```python
from build123d import *

# Parameters (mm, degrees)
SKETCH1_W          = 55
SKETCH1_H          = 55
BASE_FLANGE1_DEPTH = 0.7
EDGE_FLANGE1_DEPTH = 55
SKETCH10_R         = 2
CUT_EXTRUDE1_DEPTH = 10


# Sheet-metal steps are written as plain solids
with BuildPart() as part:
    # Sketch1 → Base-Flange1 (new body)
    with BuildSketch(Plane.XY):
        Rectangle(SKETCH1_W, SKETCH1_H)
    extrude(amount=-BASE_FLANGE1_DEPTH)

    # Edge-Flange1 section (across the edge) → Edge-Flange1 (add)
    with BuildSketch(Plane(origin=(-27.5, 27.914213562, -0.7), x_dir=(0, -0.7071067811865438, -0.7071067811865512), z_dir=(1, 0, 0))):
        with BuildLine():
            Line((-0.7, 0.414213562), (-0.7, 54.710050506))
            Line((-0.7, 54.710050506), (0, 54.710050506))
            Line((0, 54.710050506), (0, 0.414213562))
            ThreePointArc((0, 0.414213562), (0.076120467, 0.03153013), (0.292893219, -0.292893219))
            Line((0.292893219, -0.292893219), (-0.202081528, -0.787867966))
            ThreePointArc((-0.202081528, -0.787867966), (-0.570595205, -0.236348273), (-0.7, 0.414213562))
        make_face()
    extrude(amount=EDGE_FLANGE1_DEPTH)

    # Sketch10 → Cut-Extrude1 (cut)
    with BuildSketch(Plane.XY):
        Circle(SKETCH10_R)
    extrude(amount=-CUT_EXTRUDE1_DEPTH, mode=Mode.SUBTRACT)


solid = part.part
```
Verification items for the finished model (mm, model axes). A direction names the side the tool comes from. Coordinates: 2 decimals unless noted, no trailing zeros. Loops run counter-clockwise (first coordinate to the right, second up) from the corner with the lowest first, then second, coordinate; pieces in that order, holes last. Notation, with made-up numbers: (83, 0.25) -> (111, 0.25) arc R26 ccw to (111, 19.25) -> close; hole circle Ø5 at (-24.75, -26). An arc over 180 degrees is marked (long way). Answer in a Markdown table with one row per item. Add a question column.
1. Section check B-B, the plane x = 0. Enter the section's corners in (y, z), then the cut area to 3 significant figures.
2. Draft check along Y on faces 3 (the face through (-0.434, -1.952, -0.345)), 4 (the face through (-0.385, 47.672, -20.458)), 5 (the face through (-0.385, 47.63, -19.426)). Enter one of: +Y half, -Y half, draft (parallel to the pull), parting line (faces both ways), or undercut.
3. Section check D-D, the plane y = 12.5. Enter the section's corners in (x, z), then the cut area to 3 significant figures.
4. Access from +Z, -Z, +X, -X, +Y, -Y to the whole of each face (thin tool, end or side, straight path). Record for faces 1 (the face through (0, 6, 0)), 2 (the face through (0, 6, -0.7)).
5. Depth check by flat-ended pin: P1, Ø10, axis at x = 6.5, y = 31.5, coming from the -Z side; P2, Ø6, axis at x = 4, z = -12, coming from the -Y side; P3, Ø1, axis at x = 7.5, y = -14, coming from the -Z side. Enter the tip coordinate at first touch or a pass-through.
6. Section check A-A, the plane y = 0. Enter the section's corners in (x, z).
7. Section check C-C, the plane x = 20.5. Enter the section's corners in (y, z).
8. Material ranges on probe 1 along Y at (x, z) = (0, -0.5); probe 2 along Z at (x, y) = (-22, -11.5); probe 3 along Y at (x, z) = (0, -0.2), recorded low to high. Write a range as [from, to].
Derived:
| question | item | result |
|---|---|---|
| 1 | outline | (-27.5, -0.7) -> (-2, -0.7) -> (-2, 0) -> (-27.5, 0) -> close; (2, -0.7) -> (27.5, -0.7) arc R1 cw to (28.21, -0.99) -> (66.6, -39.39) -> (67.1, -38.89) -> (28.7, -0.5) arc R1.7 ccw to (27.5, 0) -> (2, 0) -> close |
| 1 | area | 74.4 mm² |
| 2 | face 3 | undercut |
| 2 | face 4 | -Y half |
| 2 | face 5 | +Y half |
| 3 | outline | (-27.5, -0.7) -> (27.5, -0.7) -> (27.5, 0) -> (-27.5, 0) -> close |
| 3 | area | 38.5 mm² |
| 4 | face 1 | +Z, +X, -X, +Y, -Y |
| 4 | face 2 | -Z, +X, -X, -Y |
| 5 | P1 | stops at z = -9.29 |
| 5 | P2 | stops at y = 36.21 |
| 5 | P3 | stops at z = -0.7 |
| 6 | outline | (-27.5, -0.7) -> (-2, -0.7) -> (-2, 0) -> (-27.5, 0) -> close; (2, -0.7) -> (27.5, -0.7) -> (27.5, 0) -> (2, 0) -> close |
| 7 | outline | (-27.5, -0.7) -> (27.5, -0.7) arc R1 cw to (28.21, -0.99) -> (66.6, -39.39) -> (67.1, -38.89) -> (28.7, -0.5) arc R1.7 ccw to (27.5, 0) -> (-27.5, 0) -> close |
| 8 | probe 1 | y = [-27.5, -2], [2, 28.7] |
| 8 | probe 2 | z = [-0.7, 0] |
| 8 | probe 3 | y = [-27.5, -2], [2, 28.3] |
